Build history of the part. All positions in model axes, mm. Give positions to 0.01 mm unless a question says otherwise; leave off trailing zeros. Loops run counter-clockwise (first coordinate to the right, second up) from the corner with the lowest first, then second, coordinate; pieces in that order, holes last. Notation, with made-up numbers: M 2.5,-28.5 L 45.5,-28.5 A24 ccw 45.5,9.5 Z; hole C -27,29.5 d1. An arc over 180 degrees is marked long. Answer in a Markdown table with one row per item. Add a question column.
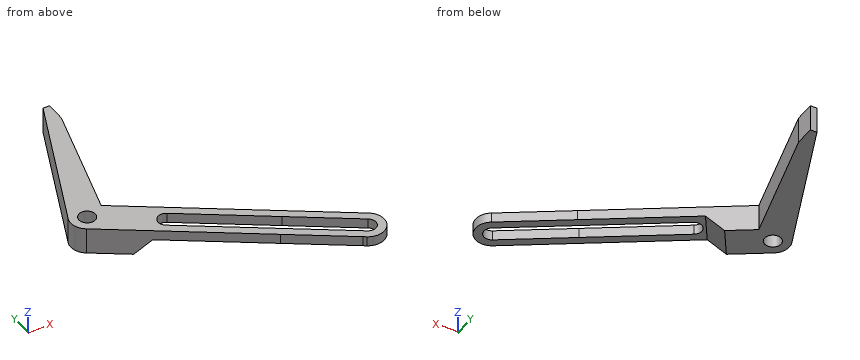
Autodesk Inventor part; units mm, degrees
ref_plane "YZ Plane" through (0, 0, 0) normal (1, 0, 0) x (0, 1, 0)
ref_plane "XZ Plane" through (0, 0, 0) normal (0, 1, 0) x (-1, 0, 0)
ref_plane "XY Plane" through (0, 0, 0) normal (0, 0, 1) x (1, 0, 0)
sketch "Sketch2" plane through (0, 0, 0) normal (0, 0, 1) x (1, 0, 0)
  line L0 (-27, 0) -> (18, 0) construction
  circle A0 centre (-42.3909, -42.2862) radius 2.5
  line L1 (-1.368, -72.0925) -> (-26.478, -55.6764)
  arc A1 (-23.742, -51.4914) -> (-26.478, -55.6764) centre (-25.11, -53.5839) ccw
  line L2 (-23.742, -51.4914) -> (1.368, -67.9075)
  arc A2 (-47.0093, -40.3702) -> (-45.1269, -46.4712) centre (-42.3909, -42.2862) ccw
  line L3 (-27, 0) -> (-27, 3)
  line L4 (-27, 3) -> (-27, -3)
  line L5 (-29.0168, 3) -> (-27, 3)
  line L6 (-27, 3) -> (-27, -3)
  line L7 (-29.0168, 3) -> (-47.0093, -40.3702)
  line L8 (-27, -3) -> (-36.781, -39.9801)
  line L9 (-45.1269, -46.4712) -> (-2.736, -74.185)
  line L10 (-36.781, -39.9801) -> (2.736, -65.815)
  line L11 (-2.736, -74.185) -> (15.2131, -85.9196)
  line L12 (2.736, -65.815) -> (21.5936, -78.1435)
  line L13 (15.2131, -85.9196) -> (16.1216, -86.5135)
  arc A3 (16.1216, -86.5135) -> (21.5936, -78.1435) centre (18.8576, -82.3285) ccw
  line L14 (1.368, -67.9075) -> (20.2256, -80.236)
  line L15 (17.4896, -84.421) -> (-1.368, -72.0925)
  arc A4 (17.4896, -84.421) -> (20.2256, -80.236) centre (18.8576, -82.3285) ccw
  point P0 (0, 0)
extrude "Extrusion2" add sketch "Sketch2" along normal blind 8
sketch "Sketch3" plane through (-36.781, -39.9801, 8) normal (0.5472037, 0.8369994, 0) x (0.8369994, -0.5472037, 0)
  line L0 (74.7426, 8) -> (74.7426, 0)
  line L1 (8.9084, 8) -> (74.7426, 8)
  line L2 (74.7426, 8) -> (74.7426, 3)
  line L3 (74.7426, 3) -> (13.9084, 3)
  line L4 (8.9084, 8) -> (13.9084, 3)
  line L5 (8.9084, 8) -> (15.9795, 8) construction
  point P0 (74.7426, 8)
  dimension "d30" = 5
  dimension "d31" = 45
extrude "Extrusion3" cut sketch "Sketch3" against normal blind 10
properties part number "Sliding linkage"
(1) Slice it at A-A, the plane x = 18.5. Give the cut face in (y, z).
(2) Slice it at C-C, the plane y = -59. Give the cut face in (x, z), then the cut area to 3 significant figures.
(3) Wall check: line 1 (X direction, y = -54, z = 7.25); line 2 (Y direction, x = -10, z = 5.75); line 3 (X direction, y = -72, z = 7.5). Give the ranges that are in metal, low to high.
(4) Slice it at D-D, the plane y = -22. Give the cut face in (x, z), then the cut area to 3 significant figures.
(5) Pin check, flat tips, straight feed: pin 1 (6 mm diameter, centred on x = -42.39, y = -42.29, fed in from -Z); pin 2 (3 mm diameter, centred on y = 0, z = 4.5, fed in from +X); pin 3 (12 mm diameter, centred on x = -8, y = -72, fed in from -Z); pin 4 (12 mm diameter, centred on x = -15.5, y = -46.5, fed in from -Z). Stop position of each tip, or through.
(6) Slice it at B-B, the plane z = 1.5. Give the cut face in (x, y).
Solution:
| question | item | result |
|---|---|---|
| 1 | outline | M -87.32,5 L -84.8,5 L -84.8,8 L -87.32,8 Z; M -79.11,5 L -76.12,5 L -76.12,8 L -79.11,8 Z |
| 2 | outline | M -25.96,5 L -21.39,5 L -21.39,8 L -25.96,8 Z; M -12.26,5 L -7.69,5 L -7.69,8 L -12.26,8 Z |
| 2 | area | 27.4 mm^2 |
| 3 | line 1 | -33.61 to -27.58, -19.9 to -15.34 |
| 3 | line 2 | -69.44 to -66.45, -60.48 to -57.49 |
| 3 | line 3 | -6.08 to -1.51, 7.63 to 12.2 |
| 4 | outline | M -39.39,0 L -32.03,0 L -32.03,8 L -39.39,8 Z |
| 4 | area | 58.9 mm^2 |
| 5 | pin 1 | z = 0 |
| 5 | pin 2 | x = -27 |
| 5 | pin 3 | z = 5 |
| 5 | pin 4 | through |
| 6 | outline | M -47.01,-40.37 A5 ccw -45.13,-46.47 L -33.54,-54.05 L -28.07,-45.68 L -36.78,-39.98 L -27,-3 L -27,3 L -29.02,3 Z; hole C -42.39,-42.29 d5 |
